Geometry check sheet. Reference: the model listing, model coordinates, mm. Face numbers are marked on the shaded views. A direction names the side the tool comes from. Round coordinates to 2 decimals unless told otherwise and drop trailing zeros. Order: outer loops, then holes, each group sorted by start corner. A loop starts at its lowest first (then second) coordinate and runs counter-clockwise, first axis right, second up. Notation, with made-up numbers: (62, -18) -> (78, -18) arc R25 ccw to (78, 19) -> close; hole circle Ø8 at (-1.75, 85.5). An arc over 180 degrees is marked (long way). Use a Markdown table: item, result. Add a question column.
Item 1: Sectioned sample at A-A, the plane y = -3. Record the cut outline in (x, z), and give its area (3 significant figures).
Item 2: Sectioned sample at D-D, the plane y = 10. Record the cut outline in (x, z).
Item 3: Mould release check, pull along Y, two halves, no side actions. Record for the marked faces 1, 2 and 3: pulls with the +Y half, pulls with the -Y half, needs draft (parallel to the pull), parting line crosses it, or undercut.
Item 4: Sectioned sample at B-B, the plane x = 8.5. Record the cut outline in (y, z).
Item 5: Gauge pin test, flat ends, axial feed: pin 1 Ø0.6 at (y, z) = (-0.5, 4) entering from -X; pin 2 Ø0.6 at (y, z) = (-4, 0.5) entering from +X; pin 3 Ø1.5 at (y, z) = (14.5, 0) entering from +X. Record the tip position at first contact, or that the pin passes through.
Item 6: Set-up check for the marked faces 4, 5, 6, 7 and 8: record each of +Z, -Z, +X, -X, +Y, -Y from which the full face is reachable in a straight line by a thin tool's end or side.
Item 7: Material ranges on probe 1 along Y at (x, z) = (0, 0.55); probe 2 along Y at (x, z) = (0, 1.1); probe 3 along Z at (x, y) = (0, -3.5), recorded low to high. Write a range as [from, to].
Item 8: Sectioned sample at C-C, the plane z = 0. State how many separate pieces and enclosed holes the cut face has, and give its area (3 significant figures).
Autodesk Inventor part; units mm, degrees
ref_plane "YZ Plane" through (0, 0, 0) normal (1, 0, 0) x (0, 1, 0)
ref_plane "XZ Plane" through (0, 0, 0) normal (0, 1, 0) x (-1, 0, 0)
ref_plane "XY Plane" through (0, 0, 0) normal (0, 0, 1) x (1, 0, 0)
sketch "草圖1" plane through (0, 0, 0) normal (0, 1, 0) x (-1, 0, 0)
  line L0 (6, 2.5) -> (-6, 2.5)
  line L1 (-6, 2.5) -> (-6, -2.5)
  line L2 (-6, -2.5) -> (6, -2.5)
  line L3 (6, -2.5) -> (6, 2.5)
  line L4 (6, 2.5) -> (-6, -2.5) construction
  line L5 (-6, 2.5) -> (6, -2.5) construction
  point P0 (0, 0)
  dimension "d0" = 5
  dimension "d1" = 12
extrude "擠出1" add sketch "草圖1" along normal blind 25
sketch "草圖2" plane through (-6, 0, 2.5) normal (0, 0, 1) x (1, 0, 0)
  circle A0 centre (6, 20) radius 2.6
  circle A1 centre (6, 10) radius 2.6
  line L0 (0, 0) -> (12, 0)
  line L1 (0, 25) -> (12, 25)
  line L2 (6, 25) -> (6, 0)
  line L3 (12, 0) -> (0, 0)
  point P0 (6, 0)
  dimension "d4" = 5.2
  dimension "d5" = 5.2
  dimension "d6" = 10
  dimension "d7" = 10
  dimension "d8" = 5
extrude "擠出2" cut sketch "草圖2" against normal blind 10
sketch "草圖3" plane through (0, 0, 0) normal (0, -1, 0) x (1, 0, 0)
  circle A0 centre (0, 0) radius 5
  circle A1 centre (0, 0) radius 10
  dimension "d11" = 10
  dimension "d12" = 20
extrude "擠出3" add sketch "草圖3" along normal blind 2
sketch "草圖4" plane through (0, -2, 0) normal (0, -1, 0) x (1, 0, 0)
  circle A0 centre (0, 0) radius 6
  circle A1 centre (0, 0) radius 7
  dimension "d15" = 12
  dimension "d16" = 14
extrude "擠出4" add sketch "草圖4" along normal blind 7
sketch "草圖5" plane through (0, 0, 0) normal (0, -1, 0) x (1, 0, 0)
  line L0 (-1.5, 1) -> (1.5, 1)
  line L1 (1.5, 1) -> (1.5, -1)
  line L2 (1.5, -1) -> (-1.5, -1)
  line L3 (-1.5, -1) -> (-1.5, 1)
  line L4 (-1.5, 1) -> (1.5, -1) construction
  line L5 (1.5, 1) -> (-1.5, -1) construction
  point P0 (0, 0)
  dimension "d19" = 3
  dimension "d20" = 2
extrude "擠出5" add sketch "草圖5" along normal blind 7
sketch "草圖6" plane through (0, 0, 0) normal (0, 1, 0) x (1, 0, 0)
  line L0 (-4.3301, -2.5) -> (4.3301, -2.5)
  line L1 (-0.7875, -7.5) -> (0.7875, -7.5)
  line L2 (0.7875, -7.5) -> (0.7875, -2.5)
  line L3 (0.7875, -2.5) -> (-0.7875, -2.5)
  line L4 (-0.7875, -2.5) -> (-0.7875, -7.5)
  arc A0 (-4.3301, -2.5) -> (4.3301, -2.5) centre (0, 0) ccw
  line L5 (-0.7875, -7.5) -> (0.7875, -2.5) construction
  line L6 (0.7875, -7.5) -> (-0.7875, -2.5) construction
  line L7 (-0.7875, 7.5) -> (0.7875, 7.5)
  line L8 (0.7875, 7.5) -> (0.7875, 2.5)
  line L9 (0.7875, 2.5) -> (-0.7875, 2.5)
  line L10 (-0.7875, 2.5) -> (-0.7875, 7.5)
  arc A1 (4.3301, 2.5) -> (-4.3301, 2.5) centre (0, 0) ccw
  line L11 (-0.7875, 7.5) -> (0.7875, 2.5) construction
  line L12 (0.7875, 7.5) -> (-0.7875, 2.5) construction
  point P0 (0, -5)
  point P1 (0, 5)
extrude "擠出6" add sketch "草圖6" against normal blind 2 contours L0 L2 A0 L4 | A0 L2 L1 L4 | L7 L8 A1 L10 | A1 L8 L9 L10
sketch "草圖7" plane through (0, -9, 0) normal (0, -1, 0) x (1, 0, 0)
  circle A0 centre (0, 0) radius 6
  circle A1 centre (0, 0) radius 10
extrude "擠出7" add sketch "草圖7" along normal blind 1
sketch "草圖8" plane through (0, 0, 0) normal (0, -1, 0) x (1, 0, 0)
  line L0 (4.3301, 2.5) -> (6, 2.5)
  line L1 (-6, -2.5) -> (6, -2.5)
  line L2 (6, -2.5) -> (6, 2.5)
  line L3 (6, 2.5) -> (-6, 2.5)
  line L4 (-6, 2.5) -> (-6, -2.5)
  line L5 (-6, -2.5) -> (6, 2.5) construction
  line L6 (6, -2.5) -> (-6, 2.5) construction
  point P0 (0, 0)
extrude "擠出8" add sketch "草圖8" along normal blind 1
equation "\"d9\" = d7"
properties part number "圓形同心線圈外"
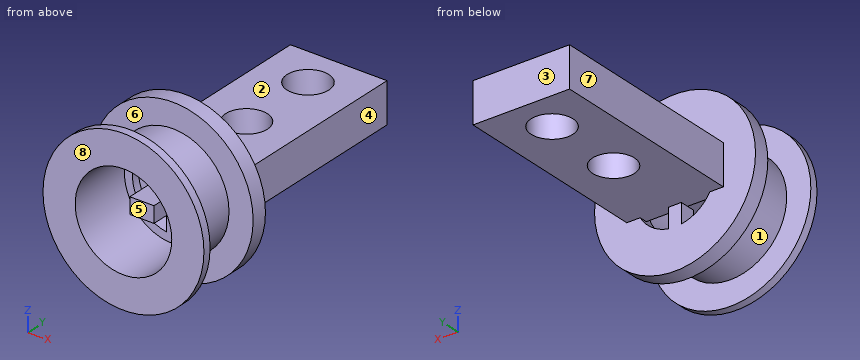
Found:
| question | item | result |
|---|---|---|
| 1 | outline | circle Ø14 at (0, 0); (-1.5, -1) -> (1.5, -1) -> (1.5, 1) -> (-1.5, 1) -> close; hole circle Ø12 at (0, 0) |
| 1 | area | 46.8 mm2 |
| 2 | outline | (-6, -2.5) -> (-2.6, -2.5) -> (-2.6, 2.5) -> (-6, 2.5) -> close; (2.6, -2.5) -> (6, -2.5) -> (6, 2.5) -> (2.6, 2.5) -> close |
| 3 | face 1 | undercut |
| 3 | face 2 | needs draft |
| 3 | face 3 | pulls with the +Y half |
| 4 | outline | (-10, -5.27) -> (-9, -5.27) -> (-9, 5.27) -> (-10, 5.27) -> close; (-2, -5.27) -> (0, -5.27) -> (0, 5.27) -> (-2, 5.27) -> close |
| 5 | pin 1 | stops at x = -9.29 |
| 5 | pin 2 | stops at x = 7 |
| 5 | pin 3 | stops at x = 6 |
| 6 | face 4 | +Z, -Z, +X, +Y |
| 6 | face 5 | -Y |
| 6 | face 6 | none |
| 6 | face 7 | +Z, -Z, -X, +Y |
| 6 | face 8 | +Z, -Z, +X, -X, -Y |
| 7 | probe 1 | y = [-7, 7.4], [12.6, 17.4], [22.6, 25] |
| 7 | probe 2 | y = [-1, 7.4], [12.6, 17.4], [22.6, 25] |
| 7 | probe 3 | z = [-7, -6], [-1, 1], [6, 7] |
| 8 | separate pieces | 1 |
| 8 | enclosed holes | 2 |
| 8 | area | 328 mm2 |
